Autodesk Inventor part; units mm, degrees
ref_plane "Work Plane1" through (29, 0, 0) normal (0, -1, 0) x (1, 0, 0)
ref_plane "YZ Plane" through (0, 0, 0) normal (1, 0, 0) x (0, 1, 0)
ref_plane "XZ Plane" through (0, 0, 0) normal (0, 1, 0) x (-1, 0, 0)
sketch "Skizze1" plane through (0, 0, 0) normal (0, 0, 1) x (1, 0, 0)
  line L0 (0.1667, 0) -> (12, 0)
  line L1 (12, 0) -> (12, 1.5)
  line L2 (12, 1.5) -> (1.5, 1.5)
  line L3 (1.5, 1.5) -> (1.1932, 1.5)
  line L4 (1.1932, 1.5) -> (0, 1.5)
  line L5 (0, 1.5) -> (0, 2.75)
  line L6 (0, 2.75) -> (-2, 2.75)
  line L7 (-2, 2.75) -> (-2, 1.1547)
  line L8 (-2, 1.1547) -> (-0.5, 1.1547)
  line L9 (-0.5, 1.1547) -> (0.1667, 0)
  line L10 (-4.8, 0) -> (14.8, 0)
  line L11 (0, -0.55) -> (0, 3.3)
  line L12 (1.5, 1.5) -> (0, 1.5) construction
  dimension "d1" = 10.5
  dimension "d2" = 0.3068
  dimension "d3" = 2
  dimension "d4" = 1.5
  dimension "d5" = 60
  dimension "d6" = 3
  dimension "d7" = 3
  dimension "d8" = 2.3094
  dimension "d9" = 5.5
  dimension "d26" = 12
revolve "Körper" add sketch "Skizze1" angle 360 about axis through (0.1667, 0, 0) along (1, 0, 0) contours L9 L11 L4 L3 L2 L1 L0 | L9 L8 L7 L6 L5 L11
sketch "Skizze2" plane through (-2, 0, 0) normal (-1, 0, 0) x (0, 0, 1)
  circle A0 centre (0, 0) radius 1.1547
  line L0 (0, -3.85) -> (0, 3.85)
  line L1 (-3.85, 0) -> (3.85, 0)
  line L2 (1.1547, 0) -> (0.5774, -1)
  line L3 (0.5774, -1) -> (-0.5774, -1)
  line L4 (-0.5774, -1) -> (-1.1547, 0)
  line L5 (-1.1547, 0) -> (-0.5774, 1)
  line L6 (-0.5774, 1) -> (0.5774, 1)
  line L7 (0.5774, 1) -> (1.1547, 0)
  point P0 (0, 0)
extrude "Loch" add sketch "Skizze2" against normal up to next contours L7 A0 | A0 L2 | L6 L0 A0 | A0 L0 L3 | L0 L6 A0 | A0 L3 L0 | L4 A0 | A0 L5
fillet "Rundung1" radius 0.3 1 edges at (-2, -2.75, 0)
thread "Gewinde"
chamfer "Fase1" distance 0.3067 distance2 0.3067 1 edges at (12, -1.5, 0) measured on face at (12, -0.6587, -0.1791)
ref_plane "Work Plane1" through (29, 0, 0) normal (0, -1, 0) x (1, 0, 0)
fillet "Fillet2" radius 0.1 1 edges at (0, -1.5, 0)
equation "\"d1\" = GEL"
equation "\"d3\" = KOH"
equation "\"d4\" = INTI"
equation "\"d6\" = GD"
equation "\"d7\" = BDM"
equation "\"d8\" = 1.1547 * SW"
equation "\"d9\" = KOD"
equation "\"d26\" = NLG"
equation "\"d30\" = R"
equation "\"d17\" = RR"
equation "\"d13\" = GEL"
equation "\"d15\" = -0.5 * SPD + 0.5 * GD"
equation "\"d16\" = GUL"
equation "\"GD\" = NND"
equation "\"NLG\" = 12"
equation "\"GEL\" = 10.5"
equation "\"KOD\" = 5.5"
equation "\"KOH\" = 2"
equation "\"INTI\" = 1.5"
equation "\"GAL\" = 0.61345 * PTC"
equation "\"GUL\" = 0.61345 * PTC"
equation "\"BDM\" = NND"
equation "\"SW\" = 2"
equation "\"RR\" = 0.3"
equation "\"SPD\" = NND - 1.2269 * PTC"
equation "\"R\" = 0.1"
equation "\"TOA\" = 30deg"
equation "\"GD1\" = THREADDIA - 1.2269 * PTC"
equation "\"THREADDIA\" = 3"
equation "\"FAWI\" = 45deg"
equation "\"ANG\" = 120deg"
equation "\"PTC\" = 0.5"
equation "\"NND\" = 3"
equation "\"E0\" = 1.155 * SW"
properties part number "DIN 7984 - M3 x 12" material "Stahl, weich"
For this review, take the finished solid that the model builds, in its own axes (mm). A direction names the side the tool comes from. Give positions to 0.01 mm unless a question says otherwise; leave off trailing zeros. Write each loop counter-clockwise with the first axis right and the second up, starting at its lowest first coordinate (ties: lowest second). Pieces come first, ordered by that corner, then holes. Notation, with made-up numbers: M 5,78.5 L 9,78.5 A18 cw 9,88.5 Z; hole C 6.5,-15.5 d4. An arc over 180 degrees is marked long. Answer as a JSON object with one key per item and string values. Group by question number.
Item 1: For probe 1 along X at (y, z) = (-1.8, -0.7); probe 2 along Y at (x, z) = (-1.5, 1.05); probe 3 along Y at (x, z) = (-0.5, -1.25), list the stretches that pass through material, from the lowest coordinate up. Write a range as [from, to].
Item 2: For pin 1 Ø2 at (x, y) = (4.5, 1) entering from -Z; pin 2 Ø2 at (x, y) = (8.5, -1) entering from +Z, all flat-tipped, find the tip position at first contact; note any pin that passes through.
Item 3: Consider section A-A on x = 10.25. Write out the cut boundary in (y, z).
Item 4: Draft analysis for pull direction Y (two halves, no side actions). For faces 1 (the cylindrical face through (-0.862, -0.596, 2.685)), 2 (the flat face through (-1.22, 0.51, 0.86)), 3 (the flat face through (-2, -1, 1)), state which applies: +Y half, -Y half, draft (parallel to the pull), parting line (faces both ways), or undercut.
Item 5: Tool access review of faces 4 (the flat face through (12, 0, 0)), 5 (the flat face through (0, 2, 0)), 6 (the flat face through (-1.22, -0.49, 0.87)): name each direction out of +Z, -Z, +X, -X, +Y, -Y from which nothing blocks a thin tool from reaching the whole face with its end or side.
Check result:
{
 "1": {"probe 1": "x = [-2, 0]", "probe 2": "y = [-2.54, -0.18], [0.18, 2.54]", "probe 3": "y = [-2.45, 2.45]"},
 "2": {"pin 1": "stops at z = -1.5", "pin 2": "stops at z = 1.5"},
 "3": {"outline": "C 0,0 d3"},
 "4": {"face 1": "parting line", "face 2": "undercut", "face 3": "draft"},
 "5": {"face 4": "+Z, -Z, +X, +Y, -Y", "face 5": "+X", "face 6": "-X"}
}
